```python
from build123d import *

# Parameters (mm, degrees)
BOSS_EXTRUDE1_DEPTH     = 5
BOSS_EXTRUDE2_DEPTH     = 5
BOSS_EXTRUDE3_DEPTH     = 5
SKETCH6_R               = 2.5
CUT_EXTRUDE1_DEPTH      = 107.549284371
SKETCH9_R               = 4.1275
SKETCH9_R_2             = 2.6035
BOSS_EXTRUDE5_DEPTH     = 35.56
FILLET1_R               = 0.508
BOSS_EXTRUDE6_DEPTH     = 19.05
SKETCH15_R              = 2.38125
BOSS_EXTRUDE7_DEPTH     = 15.875
CHAMFER2_SIZE           = 7.62
FILLET2_R               = 1.27
SKETCH16_W              = 7.844007501
SKETCH16_H              = 4.112882263
BOSS_EXTRUDE8_DEPTH     = 3.175
CHAMFER3_SIZE           = 1.27
SKETCH17_R              = 1.984375
SKETCH17_R_2            = 1.9288125
BOSS_EXTRUDE9_DEPTH     = 16.51
CUT_EXTRUDE2_REACH      = 111.603
SKETCH18_R              = 2.38125
CUT_EXTRUDE3_REACH      = 111.603
SKETCH19_R              = 2.38125
CUT_EXTRUDE4_DEPTH      = 4.13271
CUT_EXTRUDE4_DEPTH_BACK = 1.27
CUT_EXTRUDE5_DEPTH      = 1.27
SKETCH23_W              = 40.64
SKETCH23_H              = 35.56
BOSS_EXTRUDE12_DEPTH    = 5.08
CUT_EXTRUDE6_REACH      = 135.834
SKETCH24_R              = 1.7145


with BuildPart() as part:
    # Sketch1 → Boss-Extrude1 (new body)
    with BuildSketch(Plane(origin=(0, 0, 0), x_dir=(1, 0, 0), z_dir=(0, 1, 0))):
        Polygon((0, 0), (0, 60.5), (60.5, 60.5), (60.5, 47.75), (12.75, 0), align=None)
    extrude(amount=BOSS_EXTRUDE1_DEPTH)

    # Sketch4 → Boss-Extrude2 (add)
    with BuildSketch(Plane.ZY):
        Polygon((-60.5, 5), (-60.5, 68.5), (-19.4, 68.5), (0, 10.308629506), (0, 5), align=None)
    extrude(amount=-BOSS_EXTRUDE2_DEPTH)

    # Sketch5 → Boss-Extrude3 (add)
    with BuildSketch(Plane(origin=(0, 0, -60.5), x_dir=(-1, 0, 0), z_dir=(0, 0, -1))):
        Polygon((-5, 5), (-5, 68.5), (-41, 68.5), (-60.5, 10.004653177), (-60.5, 5), align=None)
    extrude(amount=-BOSS_EXTRUDE3_DEPTH)

    # Sketch6 → Cut-Extrude1 (cut, through all)
    with BuildSketch(Plane(origin=(0, 5, 0), x_dir=(1, 0, 0), z_dir=(0, 1, 0))):
        with Locations(Location((16.5, 15, 0), (0, 0, 270))):
            Circle(SKETCH6_R)
        with Locations(Location((45.5, 44.625, 0), (0, 0, 270))):
            Circle(SKETCH6_R)
    extrude(amount=-CUT_EXTRUDE1_DEPTH, mode=Mode.SUBTRACT)

    # Sketch9 → Boss-Extrude5 (add)
    with BuildSketch(Plane.XY.offset(-55.5)):
        with Locations(Location((49.45, 19.0462, 0), (0, 0, 180))):
            Circle(SKETCH9_R)
        with Locations(Location((49.45, 19.0462, 0), (0, 0, 180))):
            Circle(SKETCH9_R_2, mode=Mode.SUBTRACT)
    extrude(amount=BOSS_EXTRUDE5_DEPTH)

    # Fillet1
    fillet1_edges = [part.edges().sort_by_distance(p)[0] for p in [
        (52.0535, 19.0462, -19.94),
    ]]
    fillet(fillet1_edges, radius=FILLET1_R)

    # Sketch14 → Boss-Extrude6 (add)
    with BuildSketch(Plane(origin=(0, 5, 0), x_dir=(1, 0, 0), z_dir=(0, 1, 0))):
        with BuildLine():
            Line((6.722962691, 28.802730135), (9.132707699, 31.364136576))
            ThreePointArc((9.132707699, 31.364136576), (10.457950503, 50.042049497), (29.135863424, 51.367292301))
            Line((29.135863424, 51.367292301), (31.697269865, 53.777037309))
            ThreePointArc((31.697269865, 53.777037309), (36.686417723, 53.662894944), (36.648367319, 48.672586637))
            Line((36.648367319, 48.672586637), (33.860208422, 45.884427741))
            ThreePointArc((33.860208422, 45.884427741), (34.790141211, 43.96666613), (35.539002262, 41.971223395))
            Line((35.539002262, 41.971223395), (35.799607225, 42.077391474))
            Line((35.799607225, 42.077391474), (35.633459083, 42.367636838))
            ThreePointArc((35.633459083, 42.367636838), (35.320181387, 43.965693178), (36.041784088, 45.425561844))
            Line((36.041784088, 45.425561844), (38.110219678, 47.493997435))
            ThreePointArc((38.110219678, 47.493997435), (38.110219678, 54.843851927), (30.760365187, 54.843851927))
            Line((30.760365187, 54.843851927), (28.830026438, 52.913513178))
            ThreePointArc((28.830026438, 52.913513178), (8.980759009, 50.993661336), (7.060907167, 31.144393908))
            Line((7.060907167, 31.144393908), (5.656148073, 29.739634813))
            ThreePointArc((5.656148073, 29.739634813), (5.656148073, 22.389780322), (13.006002565, 22.389780322))
            Line((13.006002565, 22.389780322), (15.074438156, 24.458215912))
            ThreePointArc((15.074438156, 24.458215912), (15.744974902, 24.939184047), (16.534306822, 25.179818613))
            Line((16.534306822, 25.179818613), (16.568898656, 25.694636548))
            ThreePointArc((16.568898656, 25.694636548), (15.581109404, 26.144220149), (14.615572259, 26.639791578))
            Line((14.615572259, 26.639791578), (11.827413363, 23.851632681))
            ThreePointArc((11.827413363, 23.851632681), (6.837105056, 23.813582277), (6.722962691, 28.802730135))
        make_face()
    extrude(amount=BOSS_EXTRUDE6_DEPTH)

    # Sketch15 → Boss-Extrude7 (add)
    with BuildSketch(Plane(origin=(0, 68.5, 0), x_dir=(1, 0, 0), z_dir=(0, 1, 0))):
        Polygon((5, 55.5), (5, 30.3375), (30.1625, 55.5), align=None)
        with Locations(Location((9.525, 50.975, 0), (0, 0, 270))):
            Circle(SKETCH15_R, mode=Mode.SUBTRACT)
    extrude(amount=-BOSS_EXTRUDE7_DEPTH)

    # Chamfer2
    chamfer2_edges = [part.edges().sort_by_distance(p)[0] for p in [
        (17.58125, 52.625, -42.91875),
    ]]
    chamfer(chamfer2_edges, length=CHAMFER2_SIZE)

    # Fillet2
    fillet2_edges = [part.edges().sort_by_distance(p)[0] for p in [
        (15.744974902, 5, -24.939184047),
        (14.04022036, 5, -23.423998117),
        (8.812852099, 5, -20.893477035),
        (35.320181387, 5, -43.965693178),
        (35.716533154, 5, -42.222514156),
        (37.076001883, 5, -46.45977964),
        (39.606522965, 5, -51.687147901),
    ]]
    fillet(fillet2_edges, radius=FILLET2_R)

    # Sketch16 → Boss-Extrude8 (add)
    with BuildSketch(Plane.XY.offset(-55.5)):
        with Locations((42.208447341, 21.154254949)):
            Rectangle(SKETCH16_W, SKETCH16_H)
    extrude(amount=BOSS_EXTRUDE8_DEPTH)

    # Chamfer3
    chamfer3_edges = [part.edges().sort_by_distance(p)[0] for p in [
        (38.28644359, 23.21069608, -55.07937031),
    ]]
    chamfer(chamfer3_edges, length=CHAMFER3_SIZE)

    # Sketch17 → Boss-Extrude9 (add)
    # profile 1 of 2: a face of its own
    with BuildSketch(Plane(origin=(0, 5, 0), x_dir=(1, 0, 0), z_dir=(0, 1, 0))):
        with BuildLine():
            Line((14.046968971, 26.071188289), (8.715956726, 30.921156666))
            Line((8.715956726, 30.921156666), (6.722962691, 28.802730135))
            ThreePointArc((6.722962691, 28.802730135), (6.837105056, 23.813582277), (11.827413363, 23.851632681))
            Line((11.827413363, 23.851632681), (14.046968971, 26.071188289))
        make_face()
        with Locations(Location((10.020377911, 27.007841876, 0), (0, 0, 90))):
            Circle(SKETCH17_R, mode=Mode.SUBTRACT)
    # profile 2 of 2: a face of its own
    with BuildSketch(Plane(origin=(0, 5, 0), x_dir=(1, 0, 0), z_dir=(0, 1, 0))):
        with BuildLine():
            Line((31.697269865, 53.777037309), (29.66316707, 51.863374183))
            Line((29.66316707, 51.863374183), (34.595934869, 46.620154187))
            Line((34.595934869, 46.620154187), (36.648367319, 48.672586637))
            ThreePointArc((36.648367319, 48.672586637), (36.686417723, 53.662894944), (31.697269865, 53.777037309))
        make_face()
        with Locations(Location((33.690847255, 50.732351927, 0), (0, 0, 90))):
            Circle(SKETCH17_R_2, mode=Mode.SUBTRACT)
    extrude(amount=BOSS_EXTRUDE9_DEPTH)

    # Sketch18 → Cut-Extrude2 (cut, up to next)
    with BuildSketch(Plane.ZY, mode=Mode.PRIVATE) as cut_extrude2_sk1:
        with Locations((-32.56, 49.53)):
            Circle(SKETCH18_R)
    cut_extrude2_tool1 = extrude(cut_extrude2_sk1.sketch, amount=-CUT_EXTRUDE2_REACH, mode=Mode.PRIVATE) & part.part
    add(cut_extrude2_tool1.solids().sort_by_distance((0, 49.53, -32.56))[0], mode=Mode.SUBTRACT)

    # Sketch19 → Cut-Extrude3 (cut, up to next)
    with BuildSketch(Plane(origin=(0, 0, -60.5), x_dir=(-1, 0, 0), z_dir=(0, 0, -1)), mode=Mode.PRIVATE) as cut_extrude3_sk1:
        with Locations((-27.78125, 26.19375)):
            Circle(SKETCH19_R)
    cut_extrude3_tool1 = extrude(cut_extrude3_sk1.sketch, amount=-CUT_EXTRUDE3_REACH, mode=Mode.PRIVATE) & part.part
    add(cut_extrude3_tool1.solids().sort_by_distance((27.78125, 26.19375, -60.5))[0], mode=Mode.SUBTRACT)

    # Sketch20 → Cut-Extrude4 (cut, two sides: drawn at the far end of the back side and taken through both)
    with BuildSketch(Plane.XY.offset(-55.5).offset(-CUT_EXTRUDE4_DEPTH_BACK)):
        Polygon((31.447424209, 26.19375), (29.614337105, 29.36875), (25.948162895, 29.36875), (24.115075791, 26.19375), (25.948162895, 23.01875), (29.614337105, 23.01875), align=None)
    extrude(amount=CUT_EXTRUDE4_DEPTH + CUT_EXTRUDE4_DEPTH_BACK, mode=Mode.SUBTRACT)

    # Sketch21 → Cut-Extrude5 (cut)
    with BuildSketch(Plane(origin=(5, 0, 0), x_dir=(0, 0, -1), z_dir=(1, 0, 0))):
        Polygon((34.393087105, 52.705), (30.726912895, 52.705), (28.893825791, 49.53), (30.726912895, 46.355), (34.393087105, 46.355), (36.226174209, 49.53), align=None)
    extrude(amount=-CUT_EXTRUDE5_DEPTH, mode=Mode.SUBTRACT)

    # Sketch23 → Boss-Extrude12 (add)
    with BuildSketch(Plane(origin=(0, 0, 0), x_dir=(1, 0, 0), z_dir=(0, 1, 0))):
        with Locations((80.82, 42.72)):
            Rectangle(SKETCH23_W, SKETCH23_H)
    extrude(amount=BOSS_EXTRUDE12_DEPTH)

    # Sketch24 → Cut-Extrude6 (cut, up to next)
    with BuildSketch(Plane(origin=(0, 5.08, 0), x_dir=(1, 0, 0), z_dir=(0, 1, 0)), mode=Mode.PRIVATE) as cut_extrude6_sk1:
        with Locations(Location((65.58, 55.42, 0), (0, 0, 270))):
            Circle(SKETCH24_R)
    cut_extrude6_tool1 = extrude(cut_extrude6_sk1.sketch, amount=-CUT_EXTRUDE6_REACH, mode=Mode.PRIVATE) & part.part
    # Sketch24 → Cut-Extrude6 (cut, up to next)
    with BuildSketch(Plane(origin=(0, 5.08, 0), x_dir=(1, 0, 0), z_dir=(0, 1, 0)), mode=Mode.PRIVATE) as cut_extrude6_sk2:
        with Locations(Location((96.06, 55.42, 0), (0, 0, 270))):
            Circle(SKETCH24_R)
    cut_extrude6_tool2 = extrude(cut_extrude6_sk2.sketch, amount=-CUT_EXTRUDE6_REACH, mode=Mode.PRIVATE) & part.part
    # Sketch24 → Cut-Extrude6 (cut, up to next)
    with BuildSketch(Plane(origin=(0, 5.08, 0), x_dir=(1, 0, 0), z_dir=(0, 1, 0)), mode=Mode.PRIVATE) as cut_extrude6_sk3:
        with Locations(Location((96.06, 29.258, 0), (0, 0, 270))):
            Circle(SKETCH24_R)
    cut_extrude6_tool3 = extrude(cut_extrude6_sk3.sketch, amount=-CUT_EXTRUDE6_REACH, mode=Mode.PRIVATE) & part.part
    # Sketch24 → Cut-Extrude6 (cut, up to next)
    with BuildSketch(Plane(origin=(0, 5.08, 0), x_dir=(1, 0, 0), z_dir=(0, 1, 0)), mode=Mode.PRIVATE) as cut_extrude6_sk4:
        with Locations(Location((65.58, 29.258, 0), (0, 0, 270))):
            Circle(SKETCH24_R)
    cut_extrude6_tool4 = extrude(cut_extrude6_sk4.sketch, amount=-CUT_EXTRUDE6_REACH, mode=Mode.PRIVATE) & part.part
    add(cut_extrude6_tool1.solids().sort_by_distance((65.58, 5.08, -55.42))[0], mode=Mode.SUBTRACT)
    add(cut_extrude6_tool2.solids().sort_by_distance((96.06, 5.08, -55.42))[0], mode=Mode.SUBTRACT)
    add(cut_extrude6_tool3.solids().sort_by_distance((96.06, 5.08, -29.258))[0], mode=Mode.SUBTRACT)
    add(cut_extrude6_tool4.solids().sort_by_distance((65.58, 5.08, -29.258))[0], mode=Mode.SUBTRACT)


solid = part.part
```
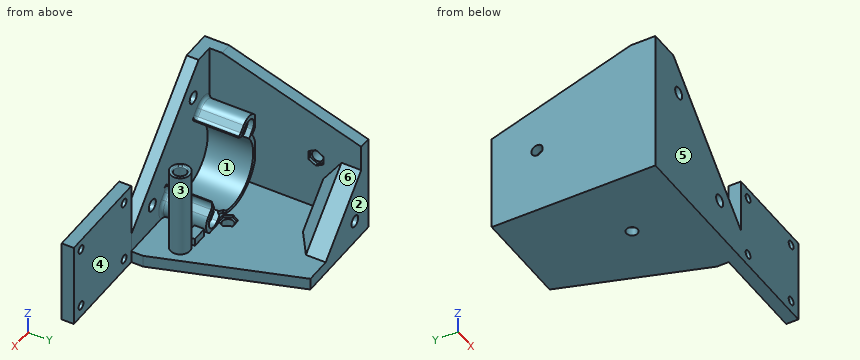
Can you work these out from the model? Positions are in its coordinate system, mm. Face numbers are marked on the shaded views. A direction names the side the tool comes from. Round coordinates to 2 decimals unless told otherwise and drop trailing zeros. Loops run counter-clockwise (first coordinate to the right, second up) from the corner with the lowest first, then second, coordinate; pieces in that order, holes last.
Item 1: Which directions (+Z, -Z, +X, -X, +Y, -Y) give clear straight access to the entire face, cutting with the end or side of a thin tool? Please do the marked faces 1 and 2.
Item 2: If we mould it in two halves opening along Y, with no side actions, what happens to the marked faces 3, 4, 5 and 6? For each: +Y half, -Y half, draft (parallel to the pull), parting line (faces both ways), or undercut.
Item 3: Please list where these lines run through material, in increasing order: L1, parallel to Y at x = 49.45, z = -27.5; L2, parallel to Y at x = 26, z = -26.
Item 4: Will these pins go through, and if not, where does the flat tip stop? pin 1 Ø3 at (x, y) = (28.5, 27) entering from +Z; pin 2 Ø4 at (x, z) = (36, -49) entering from +Y; pin 3 Ø8 at (x, z) = (16.5, -15) entering from +Y.
Item 5: Suppose I cut it at C-C, the plane y = 64. Write out the boundary of the cut face in (x, z) (1 decimal).
Item 6: Suppose I cut it at B-B, the plane z = -32.56. State how many separate pieces and enclosed holes the cut face has, then the cut area to 3 significant figures.
Item 7: Suppose I cut it at D-D, the plane z = -15. Write out the boundary of the cut face in (x, y), then the cut area to 3 significant figures.
Item 8: Suppose I cut it at A-A, the plane x = 65.58. Write out the boundary of the cut face in (y, z).
Reported:
1. face 1: none
1. face 2: +Z, -Z, +X, -X, +Y
2. face 3: undercut
2. face 4: +Y half
2. face 5: -Y half
2. face 6: draft
3. L1: y = 14.92 to 16.44, 21.65 to 23.17
3. L2: y = 0 to 5
4. pin 1: stops at z = -56.77
4. pin 2: stops at y = 24.05
4. pin 3: stops at y = 5
5. outline: (0, -60.5) - (42.5, -60.5) - (42.5, -55.5) - (30.2, -55.5) - (5, -30.3) - (5, -17.9) - (0, -17.9) - close; hole circle Ø4.8 at (9.5, -51)
6. separate pieces: 4
6. enclosed holes: 1
6. area: 817 mm2
7. outline: (0, 0) - (14, 0) - (14, 5) - (5, 5) - (5, 55.3) - (0, 55.3) - close; (19, 0) - (27.75, 0) - (27.75, 5) - (19, 5) - close
7. area: 365 mm2
8. outline: (0, -60.5) - (5.08, -60.5) - (5.08, -57.13) - (0, -57.13) - close; (0, -53.71) - (5.08, -53.71) - (5.08, -30.97) - (0, -30.97) - close; (0, -27.54) - (5.08, -27.54) - (5.08, -24.94) - (0, -24.94) - close
